from build123d import *

# Parameters (mm, degrees)
SKICA1_W                 = 50
SKICA1_H                 = 65
P_IDAT_VYSUNUT_M1_DEPTH  = 20
P_IDAT_VYSUNUT_M2_DEPTH  = 50
ODEBRAT_VYSUNUT_M1_DEPTH = 5
SKICA8_R                 = 2.35
ODEBRAT_VYSUNUT_M4_DEPTH = 8.5
SKICA6_R                 = 2.8
ODEBRAT_VYSUNUT_M7_DEPTH = 10
SKICA7_R                 = 7.5
ODEBRAT_VYSUNUT_M8_DEPTH = 10


with BuildPart() as part:
    # Skica1 → Přidat vysunutím1 (new body)
    with BuildSketch(Plane.XY):
        Rectangle(SKICA1_W, SKICA1_H)
    extrude(amount=P_IDAT_VYSUNUT_M1_DEPTH)

    # Skica3 → Přidat vysunutím2 (add, through all)
    with BuildSketch(Plane(origin=(25, 0, 0), x_dir=(0, 0, -1), z_dir=(1, 0, 0))):
        Polygon((0, 32.5), (0, 48.5), (-20, 32.5), align=None)
    extrude(amount=-P_IDAT_VYSUNUT_M2_DEPTH)

    # Skica5 → Odebrat vysunutím1 (cut)
    with BuildSketch(Plane.XY.offset(20)):
        Polygon((-20.3, 31.35), (20.31, 31.35), (22.6, -31.35), (-22.6, -31.35), align=None)
    extrude(amount=-ODEBRAT_VYSUNUT_M1_DEPTH, mode=Mode.SUBTRACT)

    # Skica8 → Odebrat vysunutím4 (cut)
    with BuildSketch(Plane(origin=(0, 0, 0), x_dir=(-1, 0, 0), z_dir=(0, 0, -1))):
        with Locations((7.14901322, 24.75)):
            Circle(SKICA8_R)
        with Locations(Location((-7.14901322, 24.75, 0), (0, 0, 180))):
            Circle(SKICA8_R)
        with Locations(Location((7.14901322, 39.05, 0), (0, 0, 180))):
            Circle(SKICA8_R)
        with Locations((-7.14901322, 39.05)):
            Circle(SKICA8_R)
    extrude(amount=-ODEBRAT_VYSUNUT_M4_DEPTH, mode=Mode.SUBTRACT)

    # Skica6 → Odebrat vysunutím7 (cut)
    with BuildSketch(Plane.XY.offset(15)):
        with Locations((0, -2.15)):
            Circle(SKICA6_R)
    extrude(amount=-ODEBRAT_VYSUNUT_M7_DEPTH, mode=Mode.SUBTRACT)

    # Skica7 → Odebrat vysunutím8 (cut)
    with BuildSketch(Plane(origin=(0, 0, 0), x_dir=(-1, 0, 0), z_dir=(0, 0, -1))):
        with Locations((0, -2.15)):
            Circle(SKICA7_R)
    extrude(amount=-ODEBRAT_VYSUNUT_M8_DEPTH, mode=Mode.SUBTRACT)


solid = part.part
Source: CAD feature listing. Evaluate the final solid. Frame: model axes, mm. A direction names the side the tool comes from. Round coordinates to 2 decimals unless told otherwise and drop trailing zeros. Loops run counter-clockwise (first coordinate to the right, second up) from the corner with the lowest first, then second, coordinate; pieces in that order, holes last. Notation, with made-up numbers: (-35, 13) -> (19, 13) arc R24 cw to (19, 32) -> close; hole circle Ø11 at (-35, 30). An arc over 180 degrees is marked (long way). Answer as a JSON object with one key per item and string values. Group by question number.
Q1. Contact query for flat-ended pins moving along their axis: P1, Ø4, axis at x = 7.15, y = 39.05, coming from the -Z side; P2, Ø24, axis at x = 0, y = -2.15, coming from the +Z side; P3, Ø5, axis at x = 6.5, y = 24.5, coming from the -Z side; P4, Ø5.5, axis at x = 6, z = 18.5, coming from the +Y side. Output: stop coordinate, or through.
Q2. Access query for faces 1 (the flat face through (7, 25, 8.5)), 2 (the flat face through (-21.466, -0.439, 17.535)), 3 (the flat face through (-22, 7, 20)). Directions: +Z, -Z, +X, -X, +Y, -Y. A direction counts if a zero-diameter tool reaches every point of the face in a straight line with its end or side. Return the directions, or none.
Q3. Section query C-C (z = 16.75). Output: boundary loops of the cut face in (x, y), plus the area to 3 significant figures.
Q4. Ray query, line 1 (X direction, y = 24.5, z = 6); line 2 (Z direction, x = 5, y = 36.5); line 3 (Y direction, x = 0.5, z = 17.25). Return the intervals inside material, ascending. Write a range as from..to.
Q5. Mould query, pull axis X, two halves, no side actions, for faces 4 (the flat face through (-25, 9, 10)), 5 (the flat face through (0.35, 40.61, 9.86)), 6 (the cylindrical face through (-8.233, 22.665, 4.19)), 7 (the flat face through (25, 9, 10)). Classes: pulls with the +X half, pulls with the -X half, needs draft (parallel to the pull), parting line crosses it, or undercut.
Q6. Section query A-A (x = 0). Output: boundary loops of the cut face in (y, z).
Q7. Section query D-D (y = -2.15). Output: boundary loops of the cut face in (x, z), plus the area to 3 significant figures.
Q8. Section query B-B (z = 5.75). Output: boundary loops of the cut face in (x, y), plus the area to 3 significant figures.
Completed:
{
 "1": {"P1": "z = 8.5", "P2": "z = 15", "P3": "z = 0", "P4": "y = 35.9"},
 "2": {"face 1": "-Z", "face 2": "+Z", "face 3": "+Z, +X, -X, +Y, -Y"},
 "3": {"outline": "(-25, -32.5) -> (25, -32.5) -> (25, 35.1) -> (-25, 35.1) -> close; hole (-22.6, -31.35) -> (22.6, -31.35) -> (20.31, 31.35) -> (-20.3, 31.35) -> close", "area": "690 mm²"},
 "4": {"line 1": "-25..-9.49, -4.81..4.81, 9.49..25", "line 2": "0..15", "line 3": "-32.5..-31.35, 31.35..34.7"},
 "5": {"face 4": "pulls with the -X half", "face 5": "needs draft", "face 6": "undercut", "face 7": "pulls with the +X half"},
 "6": {"outline": "(-32.5, 0) -> (-9.65, 0) -> (-9.65, 10) -> (-4.95, 10) -> (-4.95, 15) -> (-31.35, 15) -> (-31.35, 20) -> (-32.5, 20) -> close; (0.65, 10) -> (5.35, 10) -> (5.35, 0) -> (48.5, 0) -> (32.5, 20) -> (31.35, 20) -> (31.35, 15) -> (0.65, 15) -> close"},
 "7": {"outline": "(-25, 0) -> (-7.5, 0) -> (-7.5, 10) -> (-2.8, 10) -> (-2.8, 15) -> (-21.53, 15) -> (-21.53, 20) -> (-25, 20) -> close; (2.8, 10) -> (7.5, 10) -> (7.5, 0) -> (25, 0) -> (25, 20) -> (21.53, 20) -> (21.53, 15) -> (2.8, 15) -> close", "area": "607 mm²"},
 "8": {"outline": "(-25, -32.5) -> (25, -32.5) -> (25, 43.9) -> (-25, 43.9) -> close; hole circle Ø4.7 at (-7.15, 24.75); hole circle Ø4.7 at (-7.15, 39.05); hole circle Ø15 at (0, -2.15); hole circle Ø4.7 at (7.15, 24.75); hole circle Ø4.7 at (7.15, 39.05)", "area": "3,570 mm²"}
}
